from build123d import *

# Parameters (mm, degrees)
SKETCH1_W               = 151
SKETCH1_H               = 49
BOSS_EXTRUDE1_DEPTH     = 49
SKETCH2_W               = 51.3
SKETCH2_H               = 41.9
CUT_EXTRUDE1_DEPTH      = 4.2596
CUT_EXTRUDE2_DEPTH      = 103.480485947
CUT_EXTRUDE2_DEPTH_BACK = 103.480485947


with BuildPart() as part:
    # Sketch1 → Boss-Extrude1 (new body)
    with BuildSketch(Plane(origin=(0, 0, 0), x_dir=(1, 0, 0), z_dir=(0, 1, 0))):
        Rectangle(SKETCH1_W, SKETCH1_H)
    extrude(amount=BOSS_EXTRUDE1_DEPTH)

    # Sketch2 → Cut-Extrude1 (cut)
    with BuildSketch(Plane(origin=(0, 49, 0), x_dir=(1, 0, 0), z_dir=(0, 1, 0))):
        with Locations((45.324412799, 0)):
            Rectangle(SKETCH2_W, SKETCH2_H)
    extrude(amount=-CUT_EXTRUDE1_DEPTH, mode=Mode.SUBTRACT)

    # Sketch6 → Cut-Extrude2 (cut, two sides: drawn at the far end of the back side and taken through both)
    with BuildSketch(Plane(origin=(0, 0, -24.5), x_dir=(-1, 0, 0), z_dir=(0, 0, -1)).offset(-CUT_EXTRUDE2_DEPTH_BACK)):
        with BuildLine():
            Line((-63.774014365, 48.05), (-63.774014365, 49))
            ThreePointArc((-63.774014365, 49), (-60.574014365, 52.2), (-57.374014365, 49))
            Line((-57.374014365, 49), (-57.374014365, 48.05))
            ThreePointArc((-57.374014365, 48.05), (-60.574014365, 44.85), (-63.774014365, 48.05))
        make_face()
    extrude(amount=CUT_EXTRUDE2_DEPTH + CUT_EXTRUDE2_DEPTH_BACK, mode=Mode.SUBTRACT)


solid = part.part
Work out the finished part from the listing and answer in its coordinate system (mm). A direction names the side the tool comes from. Give positions to 0.01 mm unless a question says otherwise; leave off trailing zeros. Write each loop counter-clockwise with the first axis right and the second up, starting at its lowest first coordinate (ties: lowest second). Pieces come first, ordered by that corner, then holes. Notation, with made-up numbers: (-4.75, -5.5) - (31.25, -5.5) arc R34 cw to (31.25, 27.5) - close; hole circle Ø5 at (68.5, -1). An arc over 180 degrees is marked (long way). One line per item, written item: value. Start each with the question number.
1. For a pull along X with two mould halves and no side action, classify faces 1 (the flat face through (45, 47, -20.95)), 2 (the flat face through (-1, 24, 24.5)), 3 (the flat face through (-75.5, 24, 0)) as +X half, -X half, draft (parallel to the pull), parting line (faces both ways), or undercut.
2. Consider probe 1 along X at (y, z) = (46, 11.5); probe 2 along Y at (x, z) = (57, -13). Determine where each line is inside the solid, lowest interval first.
3. Find section A-A (z = -16.5). Write down the section's boundary in (x, y).
4. For faces 4 (the flat face through (-1, 0, 0)), 5 (the flat face through (70.974, 47, 0)), determine the directions among +Z, -Z, +X, -X, +Y, -Y from which every point of the face is accessible in a straight line to the end or side of a thin tool.
Geometry results:
1. face 1: undercut
1. face 2: draft
1. face 3: -X half
2. probe 1: -75.5 to 19.67, 70.97 to 75.5
2. probe 2: 0 to 44.74
3. outline: (-75.5, 0) - (75.5, 0) - (75.5, 49) - (70.97, 49) - (70.97, 44.74) - (19.67, 44.74) - (19.67, 49) - (-75.5, 49) - close
4. face 4: +Z, -Z, +X, -X, -Y
4. face 5: +Y
